```python
from build123d import *

# Parameters (mm, degrees)
SKETCH1_W           = 80
SKETCH1_H           = 140
BOSS_EXTRUDE1_DEPTH = 3
SKETCH2_W           = 80
SKETCH2_H           = 140
SKETCH2_W_2         = 74
SKETCH2_H_2         = 134
BOSS_EXTRUDE2_DEPTH = 60
FILLET1_R           = 2
FILLET2_R           = 2
SKETCH6_W           = 80
SKETCH6_H           = 140
BOSS_EXTRUDE3_DEPTH = 12
CUT_EXTRUDE1_DEPTH  = 3
SKETCH8_R           = 1.15
CUT_EXTRUDE2_DEPTH  = 6
FILLET3_R           = 3
SKETCH9_W           = 5
SKETCH9_H           = 30
BOSS_EXTRUDE4_DEPTH = 15
SKETCH10_W          = 5
SKETCH10_H          = 30
BOSS_EXTRUDE5_DEPTH = 53
FILLET4_R           = 3
FILLET5_R           = 3
SKETCH12_W          = 5
SKETCH12_H          = 10
BOSS_EXTRUDE6_DEPTH = 19.88
FILLET6_R           = 2
FILLET7_R           = 2
SKETCH13_R          = 1.9
CUT_EXTRUDE3_DEPTH  = 172.800029104
SKETCH14_W          = 8.2
SKETCH14_H          = 3
CUT_EXTRUDE4_DEPTH  = 3
BOSS_EXTRUDE7_DEPTH = 1.35
SKETCH16_W          = 5
SKETCH16_H          = 2.7
CUT_EXTRUDE5_DEPTH  = 3


with BuildPart() as part:
    # Sketch1 → Boss-Extrude1 (new body)
    with BuildSketch(Plane(origin=(0, 0, 0), x_dir=(1, 0, 0), z_dir=(0, 1, 0))):
        with Locations((40, 70)):
            Rectangle(SKETCH1_W, SKETCH1_H)
    extrude(amount=BOSS_EXTRUDE1_DEPTH)

    # Sketch2 → Boss-Extrude2 (add)
    with BuildSketch(Plane(origin=(0, 3, 0), x_dir=(1, 0, 0), z_dir=(0, 1, 0))):
        with Locations((40, 70)):
            Rectangle(SKETCH2_W, SKETCH2_H)
        with Locations((40, 70)):
            Rectangle(SKETCH2_W_2, SKETCH2_H_2, mode=Mode.SUBTRACT)
    extrude(amount=BOSS_EXTRUDE2_DEPTH)

    # Fillet1
    fillet1_edges = [part.edges().sort_by_distance(p)[0] for p in [
        (3, 3, -70),
        (40, 3, -3),
        (77, 3, -70),
        (40, 3, -137),
        (3, 33, -3),
        (77, 33, -3),
        (77, 33, -137),
        (3, 33, -137),
    ]]
    fillet(fillet1_edges, radius=FILLET1_R)

    # Fillet2
    fillet2_edges = [part.edges().sort_by_distance(p)[0] for p in [
        (40, 0, -140),
        (80, 0, -70),
        (40, 0, 0),
        (0, 0, -70),
    ]]
    fillet(fillet2_edges, radius=FILLET2_R)

    # Sketch6 → Boss-Extrude3 (add)
    with BuildSketch(Plane(origin=(0, 63, 0), x_dir=(1, 0, 0), z_dir=(0, 1, 0))):
        with Locations((40, 70)):
            Rectangle(SKETCH6_W, SKETCH6_H)
        with BuildLine():
            Line((15, 128), (65, 128))
            ThreePointArc((65, 128), (67.121320344, 127.121320344), (68, 125))
            Line((68, 125), (68, 15))
            ThreePointArc((68, 15), (67.121320344, 12.878679656), (65, 12))
            Line((65, 12), (15, 12))
            ThreePointArc((15, 12), (12.878679656, 12.878679656), (12, 15))
            Line((12, 15), (12, 125))
            ThreePointArc((12, 125), (12.878679656, 127.121320344), (15, 128))
        make_face(mode=Mode.SUBTRACT)
    extrude(amount=BOSS_EXTRUDE3_DEPTH)

    # Sketch7 → Cut-Extrude1 (cut)
    with BuildSketch(Plane(origin=(0, 75, 0), x_dir=(1, 0, 0), z_dir=(0, 1, 0))):
        with BuildLine():
            Line((6, 137), (74, 137))
            ThreePointArc((74, 137), (76.121320344, 136.121320344), (77, 134))
            Line((77, 134), (77, 6))
            ThreePointArc((77, 6), (76.121320344, 3.878679656), (74, 3))
            Line((74, 3), (6, 3))
            ThreePointArc((6, 3), (3.878679656, 3.878679656), (3, 6))
            Line((3, 6), (3, 134))
            ThreePointArc((3, 134), (3.878679656, 136.121320344), (6, 137))
        make_face()
        with BuildLine():
            Line((12, 131), (68, 131))
            ThreePointArc((68, 131), (70.121320344, 130.121320344), (71, 128))
            Line((71, 128), (71, 12))
            ThreePointArc((71, 12), (70.121320344, 9.878679656), (68, 9))
            Line((68, 9), (12, 9))
            ThreePointArc((12, 9), (9.878679656, 9.878679656), (9, 12))
            Line((9, 12), (9, 128))
            ThreePointArc((9, 128), (9.878679656, 130.121320344), (12, 131))
        make_face(mode=Mode.SUBTRACT)
    extrude(amount=-CUT_EXTRUDE1_DEPTH, mode=Mode.SUBTRACT)

    # Sketch8 → Cut-Extrude2 (cut)
    with BuildSketch(Plane(origin=(0, 72, 0), x_dir=(1, 0, 0), z_dir=(0, 1, 0))):
        with Locations(Location((6.5, 6.5, 0), (0, 0, 270))):
            Circle(SKETCH8_R)
        with Locations(Location((73.5, 6.5, 0), (0, 0, 270))):
            Circle(SKETCH8_R)
        with Locations(Location((73.5, 133.5, 0), (0, 0, 270))):
            Circle(SKETCH8_R)
        with Locations(Location((6.5, 133.5, 0), (0, 0, 270))):
            Circle(SKETCH8_R)
    extrude(amount=-CUT_EXTRUDE2_DEPTH, mode=Mode.SUBTRACT)

    # Fillet3
    # the kernel refuses this fillet: 3 mm, written as the material it takes off along each edge
    with BuildSketch(Plane(origin=(77, 0, -3), x_dir=(1, 0, 0), z_dir=(0, 0, -1))) as fillet3_piece_1:
        with BuildLine():
            CenterArc((1, -2), 2, 0, 90)
            Line((3, -2), (3, 0))
            Line((3, 0), (1, 0))
        make_face()
    revolve(axis=Axis((77, 0, -3), (0, -1, 0)), revolution_arc=90, mode=Mode.SUBTRACT)
    with BuildSketch(Plane(origin=(3, 0, -3), x_dir=(0, 0, 1), z_dir=(1, 0, 0))) as fillet3_piece_2:
        with BuildLine():
            CenterArc((1, -2), 2, 0, 90)
            Line((3, -2), (3, 0))
            Line((3, 0), (1, 0))
        make_face()
    revolve(axis=Axis((3, 0, -3), (0, -1, 0)), revolution_arc=90, mode=Mode.SUBTRACT)
    with BuildSketch(Plane(origin=(77, 0, -137), x_dir=(0, 0, -1), z_dir=(-1, 0, 0))) as fillet3_piece_3:
        with BuildLine():
            CenterArc((1, -2), 2, 0, 90)
            Line((3, -2), (3, 0))
            Line((3, 0), (1, 0))
        make_face()
    revolve(axis=Axis((77, 0, -137), (0, -1, 0)), revolution_arc=90, mode=Mode.SUBTRACT)
    with BuildSketch(Plane(origin=(3, 0, -137), x_dir=(-1, 0, 0), z_dir=(0, 0, 1))) as fillet3_piece_4:
        with BuildLine():
            CenterArc((1, -2), 2, 0, 90)
            Line((3, -2), (3, 0))
            Line((3, 0), (1, 0))
        make_face()
    revolve(axis=Axis((3, 0, -137), (0, -1, 0)), revolution_arc=90, mode=Mode.SUBTRACT)
    with BuildSketch(Plane(origin=(0, 0, -140), x_dir=(1, 0, 0), z_dir=(0, 1, 0)), Plane(origin=(80, 82.5, -140), x_dir=(-1, 0, 0), z_dir=(0, -1, 0)), Plane(origin=(80, 82.5, 0), x_dir=(0, 0, -1), z_dir=(0, -1, 0)), Plane(origin=(0, 0, 0), x_dir=(0, 0, -1), z_dir=(0, 1, 0))) as fillet3_piece_5:
        with BuildLine():
            CenterArc((FILLET3_R, -FILLET3_R), FILLET3_R, 90, 90)
            Line((0, -FILLET3_R), (0, 0))
            Line((0, 0), (FILLET3_R, 0))
        make_face()
    extrude(amount=82.5, mode=Mode.SUBTRACT)

    # Sketch9 → Boss-Extrude4 (add)
    with BuildSketch(Plane.ZY):
        with Locations((-84.5, 40)):
            Rectangle(SKETCH9_W, SKETCH9_H)
    extrude(amount=BOSS_EXTRUDE4_DEPTH)

    # Sketch10 → Boss-Extrude5 (add)
    with BuildSketch(Plane(origin=(0, 0, -87), x_dir=(-1, 0, 0), z_dir=(0, 0, -1))):
        with Locations((12.5, 40)):
            Rectangle(SKETCH10_W, SKETCH10_H)
    extrude(amount=BOSS_EXTRUDE5_DEPTH)

    # Fillet4
    fillet4_edges = [part.edges().sort_by_distance(p)[0] for p in [
        (0, 40, -87),
        (0, 25, -84.5),
        (0, 40, -82),
        (0, 55, -84.5),
    ]]
    fillet(fillet4_edges, radius=FILLET4_R)

    # Fillet5
    fillet5_edges = [part.edges().sort_by_distance(p)[0] for p in [
        (-15, 40, -82),
        (-10, 40, -87),
        (-12.5, 55, -140),
        (-12.5, 25, -140),
    ]]
    fillet(fillet5_edges, radius=FILLET5_R)

    # Sketch12 → Boss-Extrude6 (add)
    with BuildSketch(Plane.XY):
        with Locations((17, 65)):
            Rectangle(SKETCH12_W, SKETCH12_H)
        with Locations((17, 14.67)):
            Rectangle(SKETCH12_W, SKETCH12_H)
    extrude(amount=BOSS_EXTRUDE6_DEPTH)

    # Fillet6
    fillet6_edges = [part.edges().sort_by_distance(p)[0] for p in [
        (19.5, 65, 0),
        (17, 70, 0),
        (17, 9.67, 0),
        (19.5, 14.67, 0),
    ]]
    fillet(fillet6_edges, radius=FILLET6_R)

    # Fillet7
    fillet7_edges = [part.edges().sort_by_distance(p)[0] for p in [
        (17, 60, 19.88),
        (17, 70, 19.88),
        (17, 9.67, 19.88),
        (17, 19.67, 19.88),
    ]]
    fillet(fillet7_edges, radius=FILLET7_R)

    # Sketch13 → Cut-Extrude3 (cut, through all)
    with BuildSketch(Plane.ZY.offset(-14.5)):
        with Locations(Location((4.5, 65, 0), (0, 0, 270))):
            Circle(SKETCH13_R)
        with Locations(Location((15.38, 65, 0), (0, 0, 270))):
            Circle(SKETCH13_R)
        with Locations(Location((4.5, 14.67, 0), (0, 0, 270))):
            Circle(SKETCH13_R)
        with Locations(Location((15.38, 14.67, 0), (0, 0, 270))):
            Circle(SKETCH13_R)
    extrude(amount=-CUT_EXTRUDE3_DEPTH, mode=Mode.SUBTRACT)

    # Sketch14 → Cut-Extrude4 (cut)
    with BuildSketch(Plane.XY):
        with Locations((57.9, 58.5)):
            Rectangle(SKETCH14_W, SKETCH14_H)
    extrude(amount=-CUT_EXTRUDE4_DEPTH, mode=Mode.SUBTRACT)

    # Sketch15 → Boss-Extrude7 (add)
    with BuildSketch(Plane.XZ):
        with BuildLine():
            Line((19.25, -42.75), (60.75, -42.75))
            ThreePointArc((60.75, -42.75), (61.810660172, -43.189339828), (62.25, -44.25))
            Line((62.25, -44.25), (62.25, -95.75))
            ThreePointArc((62.25, -95.75), (61.810660172, -96.810660172), (60.75, -97.25))
            Line((60.75, -97.25), (19.25, -97.25))
            ThreePointArc((19.25, -97.25), (18.189339828, -96.810660172), (17.75, -95.75))
            Line((17.75, -95.75), (17.75, -44.25))
            ThreePointArc((17.75, -44.25), (18.189339828, -43.189339828), (19.25, -42.75))
        make_face()
        with BuildLine():
            Line((21.25, -44.75), (58.75, -44.75))
            ThreePointArc((58.75, -44.75), (59.810660172, -45.189339828), (60.25, -46.25))
            Line((60.25, -46.25), (60.25, -93.75))
            ThreePointArc((60.25, -93.75), (59.810660172, -94.810660172), (58.75, -95.25))
            Line((58.75, -95.25), (21.25, -95.25))
            ThreePointArc((21.25, -95.25), (20.189339828, -94.810660172), (19.75, -93.75))
            Line((19.75, -93.75), (19.75, -46.25))
            ThreePointArc((19.75, -46.25), (20.189339828, -45.189339828), (21.25, -44.75))
        make_face(mode=Mode.SUBTRACT)
    extrude(amount=BOSS_EXTRUDE7_DEPTH)

    # Sketch16 → Cut-Extrude5 (cut)
    with BuildSketch(Plane.XZ):
        with Locations((40, -48.03)):
            Rectangle(SKETCH16_W, SKETCH16_H)
    extrude(amount=-CUT_EXTRUDE5_DEPTH, mode=Mode.SUBTRACT)


solid = part.part
```
CAD build for the part. Positions are in the model's coordinates, mm. A direction names the side the tool comes from. Round coordinates to 2 decimals unless told otherwise and drop trailing zeros. Order: outer loops, then holes, each group sorted by start corner. A loop starts at its lowest first (then second) coordinate and runs counter-clockwise, first axis right, second up.
Q1. Slice it at D-D (z = -17). Write the cut outline in (x, y), and give its area (3 significant figures).
Q2. Slice it at C-C (y = 31.5). Write the cut outline in (x, z).
Q3. Wall check: L1, parallel to Z at x = 18.4, y = 14.67; L2, parallel to X at y = 44, z = -106; L3, parallel to X at y = 70.6, z = -133.5. Give the ranges that are in metal, low to high.
Q4. Two-plate mould, pull along Y, no slides. Class faces 5 (the flat face through (73, 72, -70)), 6 (the flat face through (17, 60, 9)), 7 (the flat face through (12, 69, -69)): pulls with the +Y half, pulls with the -Y half, needs draft (parallel to the pull), parting line crosses it, or undercut.
Q5. Slice it at A-A (y = 14.67). State how many separate pieces and enclosed holes the cut face has, and give its area (3 significant figures).
Q6. Which spindle directions (+Z, -Z, +X, -X, +Y, -Y) get a long thin tool onto all of the face, cutting with end or side? Do faces 1 (the flat face through (40, 3, -71)), 2 (the flat face through (17, 70, 10)), 3 (the flat face through (17, 9.67, 10)), 4 (the flat face through (68, 69, -71)). Say none if no direction does.
Q7. Slice it at B-B (z = 15.38). Write the cut outline in (x, y), and give its area (3 significant figures).
Q8. Drop flat-ended pins along their axis: pin 1 (12 mm diameter, centred on x = 64, z = -10, fed in from -Y); pin 2 (1.2 mm diameter, centred on x = 74, z = -133, fed in from +Y); pin 3 (3 mm diameter, centred on y = 63.5, z = 11.5, fed in from +X); pin 4 (2 mm diameter, centred on y = 1, z = -47.5, fed in from +X). Give the stop position or say it passes through.
Results below:
1. outline: (0, 2) arc R2 ccw to (2, 0) - (78, 0) arc R2 ccw to (80, 2) - (80, 75) - (77, 75) - (77, 72) - (71, 72) - (71, 75) - (68, 75) - (68, 63) - (77, 63) - (77, 5) arc R2 cw to (75, 3) - (5, 3) arc R2 cw to (3, 5) - (3, 63) - (12, 63) - (12, 75) - (9, 75) - (9, 72) - (3, 72) - (3, 75) - (0, 75) - close
1. area: 852 mm2
2. outline: (-15, -140) - (-10, -140) - (-10, -90) arc R3 cw to (-7, -87) - (-3, -87) arc R3 cw to (0, -90) - (0, -137) arc R3 ccw to (3, -140) - (77, -140) arc R3 ccw to (80, -137) - (80, -3) arc R3 ccw to (77, 0) - (3, 0) arc R3 ccw to (0, -3) - (0, -79) arc R3 cw to (-3, -82) - (-12, -82) arc R3 ccw to (-15, -85) - close; hole (3, -135) arc R2 ccw to (5, -137) - (75, -137) arc R2 ccw to (77, -135) - (77, -5) arc R2 ccw to (75, -3) - (5, -3) arc R2 ccw to (3, -5) - close
3. L1: z = -140 to -137, -3 to 2.6, 6.4 to 13.48, 17.28 to 19.88
3. L2: x = -15 to -10, 0 to 3, 77 to 80
3. L3: x = 0 to 5.35, 7.65 to 72.35, 74.65 to 80
4. face 5: pulls with the +Y half
4. face 6: undercut
4. face 7: needs draft
5. separate pieces: 3
5. enclosed holes: 1
5. area: 1,340 mm2
6. face 1: none
6. face 2: +Z, +X, -X, +Y
6. face 3: +Z, +X, -X, -Y
6. face 4: +Y
7. outline: (14.5, 9.67) - (19.5, 9.67) - (19.5, 12.77) - (14.5, 12.77) - close; (14.5, 16.57) - (19.5, 16.57) - (19.5, 19.67) - (14.5, 19.67) - close; (14.5, 60) - (19.5, 60) - (19.5, 63.1) - (14.5, 63.1) - close; (14.5, 66.9) - (19.5, 66.9) - (19.5, 70) - (14.5, 70) - close
7. area: 62.0 mm2
8. pin 1: stops at y = 0
8. pin 2: stops at y = 72
8. pin 3: stops at x = 19.5
8. pin 4: stops at x = 80
